Check sheet for the modelled part. Datum: model origin and axes. Units: mm. A direction names the side the tool comes from. Coordinates: 2 decimals unless noted, no trailing zeros. Order: outer loops, then holes, each group sorted by start corner. A loop starts at its lowest first (then second) coordinate and runs counter-clockwise, first axis right, second up.
1. Gauge pin test, flat ends, axial feed: pin 1 Ø10 at (x, y) = (-12.5, -18.5) entering from -Z; pin 2 Ø1.5 at (x, y) = (-15, -4.5) entering from -Z; pin 3 Ø1.9 at (x, z) = (21, 0) entering from +Y. Record the tip position at first contact, or that the pin passes through.
2. Cross-section at B-B (y = -6). Enter the section's corners in (x, z), then the cut area to 3 significant figures.
3. Draft check along X on faces 1 (the cylindrical face through (0.39, -4.087, 4.243)), 2 (the flat face through (18, -30, -17)), 3 (the cylindrical face through (23.846, -14.79, 7.509)). Enter one of: released by +X, released by -X, zero draft, split by the parting line, or undercut.
4. Cross-section at A-A (z = 0). Count the separate pieces of the cut face and the enclosed holes in it, then the cut area to 3 significant figures.
5. Thickness scan on line 1 (Z direction, x = 0, y = -2.1); line 2 (Z direction, x = 0.5, y = -10.5) (3 decimals). Record the ranges inside material, lowest first.
6. Set-up check for faces 4 (the cylindrical face through (0.661, -1.578, 3.023)), 5 (the cylindrical face through (-4.243, -4.087, 0.39)), 6 (the cylindrical face through (-2.018, -13.902, 15.368)): record each of +Z, -Z, +X, -X, +Y, -Y from which the full face is reachable in a straight line by a thin tool's end or side.
7. Cross-section at D-D (y = -12.5). Enter the section's corners in (x, z).
```python
from build123d import *

# Parameters (mm, degrees)
SKETCH1_R           = 25
BOSS_EXTRUDE1_DEPTH = 5
SKETCH2_R           = 25
SKETCH2_R_2         = 15.5
BOSS_EXTRUDE2_DEPTH = 25
SKETCH3_R           = 3.05
SKETCH3_R_2         = 1.8
CUT_EXTRUDE1_DEPTH  = 3.2
SKETCH3_2_R         = 1.8
CUT_EXTRUDE2_DEPTH  = 5
SKETCH4_R           = 1.55
CUT_EXTRUDE4_DEPTH  = 7
CIRPATTERN1_COUNT   = 4
FILLET1_R           = 9
FILLET2_R           = 2


with BuildPart() as part:
    # Sketch1 → Boss-Extrude1 (new body)
    with BuildSketch(Plane(origin=(0, 0, 0), x_dir=(1, 0, 0), z_dir=(0, 1, 0))):
        Circle(SKETCH1_R)
    extrude(amount=-BOSS_EXTRUDE1_DEPTH)

    # Sketch2 → Boss-Extrude2 (add)
    with BuildSketch(Plane.XZ.offset(5)):
        Circle(SKETCH2_R)
        Circle(SKETCH2_R_2, mode=Mode.SUBTRACT)
    extrude(amount=BOSS_EXTRUDE2_DEPTH)

    # Sketch3 → Cut-Extrude1 (cut)
    with BuildSketch(Plane(origin=(0, 0, 0), x_dir=(1, 0, 0), z_dir=(0, 1, 0))):
        with Locations((0, 6)):
            Circle(SKETCH3_R)
        with Locations((0, 6)):
            Circle(SKETCH3_R_2, mode=Mode.SUBTRACT)
    cut_extrude1 = extrude(amount=-CUT_EXTRUDE1_DEPTH, mode=Mode.SUBTRACT)

    # Sketch3_2 → Cut-Extrude2 (cut)
    with BuildSketch(Plane(origin=(0, 0, 0), x_dir=(1, 0, 0), z_dir=(0, 1, 0))):
        with Locations((0, 6)):
            Circle(SKETCH3_2_R)
    cut_extrude2 = extrude(amount=-CUT_EXTRUDE2_DEPTH, mode=Mode.SUBTRACT)

    # Sketch4 → Cut-Extrude4 (cut)
    with BuildSketch(Plane(origin=(0, 0, 0), x_dir=(1, 0, 0), z_dir=(0, 1, 0))):
        with Locations((0, 21)):
            Circle(SKETCH4_R)
    cut_extrude4 = extrude(amount=-CUT_EXTRUDE4_DEPTH, mode=Mode.SUBTRACT)

    # CirPattern1: Cut-Extrude1, Cut-Extrude2, Cut-Extrude4 ×4 about axis
    cirpattern1_axis = Axis((0, 0, 0), (0, 1, 0))
    for i in range(1, CIRPATTERN1_COUNT):
        add(cut_extrude1.rotate(cirpattern1_axis, i * 360 / CIRPATTERN1_COUNT), mode=Mode.SUBTRACT)
        add(cut_extrude2.rotate(cirpattern1_axis, i * 360 / CIRPATTERN1_COUNT), mode=Mode.SUBTRACT)
        add(cut_extrude4.rotate(cirpattern1_axis, i * 360 / CIRPATTERN1_COUNT), mode=Mode.SUBTRACT)

    # Fillet1
    fillet1_edges = [part.edges().sort_by_distance(p)[0] for p in [
        (-15.5, -30, 0),
    ]]
    fillet(fillet1_edges, radius=FILLET1_R)

    # Fillet2
    fillet2_edges = [part.edges().sort_by_distance(p)[0] for p in [
        (-15.5, -5, 0),
    ]]
    fillet(fillet2_edges, radius=FILLET2_R)


solid = part.part
```
Data:
1. pin 1: stops at z = -23.85
1. pin 2: stops at z = -20.54
1. pin 3: stops at y = -7
2. outline: circle Ø50 at (0, 0); hole circle Ø3.1 at (-21, 0); hole circle Ø30.46 at (0, 0); hole circle Ø3.1 at (0, -21); hole circle Ø3.1 at (0, 21); hole circle Ø3.1 at (21, 0)
2. area: 1,200 mm2
3. face 1: undercut
3. face 2: zero draft
3. face 3: split by the parting line
4. separate pieces: 3
4. enclosed holes: 0
4. area: 597 mm2
5. line 1: z = -25 to -22.55, -19.45 to -9.05, -2.95 to 2.95, 9.05 to 19.45, 22.55 to 25
5. line 2: z = -24.995 to -15.492, 15.492 to 24.995
6. face 4: +Y
6. face 5: +Y, -Y
6. face 6: -Y
7. outline: circle Ø50 at (0, 0); hole circle Ø31 at (0, 0)
